Part model, mm, in its own coordinate system. A direction names the side the tool comes from. Round coordinates to 2 decimals unless told otherwise and drop trailing zeros. Order: outer loops, then holes, each group sorted by start corner. A loop starts at its lowest first (then second) coordinate and runs counter-clockwise, first axis right, second up. Notation, with made-up numbers: M 44.25,-14.75 L 66.25,-14.75 A26 cw 66.25,14.25 Z; hole C -36,-33 d4. An arc over 180 degrees is marked long. Write each question's results on one line, items separated by ' | '. Start each with the question number.
1. Band-saw the part on A-A, the plane x = 0. List the corners of the cut face in (y, z).
2. Drop flat-ended pins along their axis: pin 1 Ø3.5 at (y, z) = (-9.5, -1) entering from +X; pin 2 Ø2.5 at (x, y) = (34.43, -5) entering from +Z; pin 3 Ø0.9 at (y, z) = (-6.5, -1.5) entering from -X; pin 4 Ø8 at (x, y) = (41, 4) entering from -Z. Give the stop position or say it passes through.
3. Band-saw the part on C-C, the plane y = 16. List the corners of the cut face in (x, z).
4. Which spindle directions (+Z, -Z, +X, -X, +Y, -Y) get a long thin tool onto all of the face, cutting with end or side? Do faces 5 (the face through (44.5, 16.07, 3.54)), 6 (the face through (4.52, -13.28, -1.52)). Say none if no direction does.
5. Probe L1, parallel to Y at x = 34.43, z = 2.75; L2, parallel to Y at x = 6, z = 3.2; L3, parallel to X at y = -6, z = 5. List the from-to ranges inside material, lowest first. Write a range as [from, to].
6. Band-saw the part on B-B, the plane z = 3. Give the number of separate pieces and of enclosed holes in the cut face, then the cut area to 3 significant figures.
7. Two-plate mould, pull along X, no slides. Class faces 1 (the face through (-48, 19, 4)), 2 (the face through (50, -4, 3)), 3 (the face through (37, -4, 1)), 4 (the face through (-7, -7, 4)): +X half, -X half, draft (parallel to the pull), parting line (faces both ways), or undercut.
```python
from build123d import *

# Parameters (mm, degrees)
SKETCH_1_W                = 100
SKETCH_1_H                = 40
EXTRUDE_1_DEPTH           = 6
SKETCH_2_W                = 100
SKETCH_2_H                = 40
EXTRUDE_2_DEPTH           = 3
SKETCH_4_R                = 9.5
CUT_EXTRUDE_1_DEPTH       = 7
SKETCH_5_R                = 10.3
CUT_EXTRUDE_2_DEPTH       = 1.1
CUT_EXTRUDE_START         = -5
SKETCH_6_R                = 9.5
CUT_EXTRUDE_3_DEPTH       = 5
SKETCH_7_R                = 1.5
CUT_EXTRUDE_4_DEPTH       = 12
SKETCH_8_W                = 100
SKETCH_8_H                = 9
EXTRUDE_3_DEPTH           = 8
SKETCH_9_R                = 1.5
CUT_EXTRUDE_5_DEPTH       = 10
SKETCH_13_R               = 1.5
CUT_EXTRUDE_6_DEPTH       = 10
HOLE_WIZARD_1_D           = 3
HOLE_WIZARD_1_CBORE_D     = 5.5
HOLE_WIZARD_1_CBORE_DEPTH = 3
SKETCH_15_W               = 28
SKETCH_15_H               = 56.444719302
SKETCH_15_H_2             = 58.874458875
CUT_EXTRUDE_7_DEPTH       = 4
FILLET_3_R                = 1
FILLET_4_R                = 5
SKETCH_16_R               = 9.5
SKETCH_16_R_2             = 8.5
EXTRUDE_4_DEPTH           = 2


with BuildPart() as part:
    # 草图1 → 凸台-拉伸1 (new body)
    with BuildSketch(Plane.XY):
        Rectangle(SKETCH_1_W, SKETCH_1_H)
    extrude(amount=EXTRUDE_1_DEPTH)

    # 草图2 → 凸台-拉伸2 (add)
    with BuildSketch(Plane(origin=(0, 0, 0), x_dir=(-1, 0, 0), z_dir=(0, 0, -1))):
        Rectangle(SKETCH_2_W, SKETCH_2_H)
    extrude(amount=EXTRUDE_2_DEPTH)

    # 草图4 → 切除-拉伸1 (cut)
    with BuildSketch(Plane(origin=(0, 0, -3), x_dir=(-1, 0, 0), z_dir=(0, 0, -1))):
        Circle(SKETCH_4_R)
    extrude(amount=-CUT_EXTRUDE_1_DEPTH, mode=Mode.SUBTRACT)

    # 草图5 → 切除-拉伸2 (cut)
    with BuildSketch(Plane(origin=(0, 0, 4), x_dir=(-1, 0, 0), z_dir=(0, 0, -1))):
        Circle(SKETCH_5_R)
    extrude(amount=-CUT_EXTRUDE_2_DEPTH, mode=Mode.SUBTRACT)

    # 草图6 → 切除-拉伸3 (cut)
    with BuildSketch(Plane.XY.offset(6).offset(CUT_EXTRUDE_START)):
        with Locations(Location((0, 0, 0), (0, 0, 180))):
            Circle(SKETCH_6_R)
    extrude(amount=CUT_EXTRUDE_3_DEPTH, mode=Mode.SUBTRACT)

    # 草图7 → 切除-拉伸4 (cut)
    with BuildSketch(Plane.XY.offset(6)):
        with Locations((-15.07, 5)):
            Circle(SKETCH_7_R)
        with Locations((34.43, 5)):
            Circle(SKETCH_7_R)
        with Locations((-15.07, -5)):
            Circle(SKETCH_7_R)
        with Locations((34.43, -5)):
            Circle(SKETCH_7_R)
    extrude(amount=-CUT_EXTRUDE_4_DEPTH, mode=Mode.SUBTRACT)

    # 草图8 → 凸台-拉伸3 (add)
    with BuildSketch(Plane.XZ.offset(20)):
        with Locations((0, 1.5)):
            Rectangle(SKETCH_8_W, SKETCH_8_H)
    extrude(amount=EXTRUDE_3_DEPTH)

    # 草图9 → 切除-拉伸5 (cut)
    with BuildSketch(Plane(origin=(0, 0, -3), x_dir=(-1, 0, 0), z_dir=(0, 0, -1))):
        with Locations((-6, -15.6)):
            Circle(SKETCH_9_R)
        with Locations((6, -15.6)):
            Circle(SKETCH_9_R)
        with Locations((-16, -15.6)):
            Circle(SKETCH_9_R)
        with Locations((16, -15.6)):
            Circle(SKETCH_9_R)
    extrude(amount=-CUT_EXTRUDE_5_DEPTH, mode=Mode.SUBTRACT)

    # 草图13 → 切除-拉伸6 (cut)
    with BuildSketch(Plane.XY.offset(6)):
        with Locations((-46, 16)):
            Circle(SKETCH_13_R)
        with Locations((46, 16)):
            Circle(SKETCH_13_R)
        with Locations((-46, -24)):
            Circle(SKETCH_13_R)
        with Locations((46, -24)):
            Circle(SKETCH_13_R)
    extrude(amount=-CUT_EXTRUDE_6_DEPTH, mode=Mode.SUBTRACT)

    # 孔1 (through all)
    with Locations(Plane(origin=(-16, -15.6, -3), x_dir=(-1, 0, 0), z_dir=(0, 0, -1))):
        with Locations((0, 0), (-10, 0), (-22, 0), (-32, 0)):
            CounterBoreHole(HOLE_WIZARD_1_D / 2, HOLE_WIZARD_1_CBORE_D / 2, HOLE_WIZARD_1_CBORE_DEPTH)

    # 草图15 → 切除-拉伸7 (cut)
    with BuildSketch(Plane(origin=(0, 0, -3), x_dir=(-1, 0, 0), z_dir=(0, 0, -1))):
        with Locations((-36, -3.626193912)):
            Rectangle(SKETCH_15_W, SKETCH_15_H)
        with Locations((36, -5.588675874)):
            Rectangle(SKETCH_15_W, SKETCH_15_H_2)
    extrude(amount=-CUT_EXTRUDE_7_DEPTH, mode=Mode.SUBTRACT)

    # 圆角3
    fillet_3_edges = [part.edges().sort_by_distance(p)[0] for p in [
        (22, -4, 1),
        (-22, -4, 1),
    ]]
    fillet(fillet_3_edges, radius=FILLET_3_R)

    # 圆角4
    fillet_4_edges = [part.edges().sort_by_distance(p)[0] for p in [
        (50, -28, 3.5),
        (-50, -28, 3.5),
        (-50, 20, 3.5),
        (50, 20, 3.5),
    ]]
    fillet(fillet_4_edges, radius=FILLET_4_R)

    # 草图16 → 凸台-拉伸4 (add)
    with BuildSketch(Plane(origin=(0, 0, -3), x_dir=(-1, 0, 0), z_dir=(0, 0, -1))):
        Circle(SKETCH_16_R)
        Circle(SKETCH_16_R_2, mode=Mode.SUBTRACT)
    extrude(amount=-EXTRUDE_4_DEPTH)


solid = part.part
```
Solution:
1) outline: M -28,-3 L -8.5,-3 L -8.5,-1 L -9.5,-1 L -9.5,4 L -10.3,4 L -10.3,5.1 L -9.5,5.1 L -9.5,6 L -28,6 Z; M 8.5,-3 L 20,-3 L 20,6 L 9.5,6 L 9.5,5.1 L 10.3,5.1 L 10.3,4 L 9.5,4 L 9.5,-1 L 8.5,-1 Z
2) pin 1: x = 22.34 | pin 2: through | pin 3: x = -22 | pin 4: z = 1
3) outline: M -49.9,1 L -47.5,1 L -47.5,6 L -49.9,6 Z; M -44.5,1 L -23,1 A1 cw -22,0 L -22,-3 L 22,-3 L 22,0 A1 cw 23,1 L 44.5,1 L 44.5,6 L -44.5,6 Z; M 47.5,1 L 49.9,1 L 49.9,6 L 47.5,6 Z
4) face 5: +Z, -Z | face 6: -Z
5) L1: [-28, -6.5], [-3.5, 3.5], [6.5, 20] | L2: [-28, -17.1], [-14.1, -7.37], [7.37, 20] | L3: [-50, -16.19], [-13.95, -8.37], [8.37, 33.31], [35.55, 50]
6) separate pieces: 1 | enclosed holes: 13 | area: 4,410 mm^2
7) face 1: -X half | face 2: +X half | face 3: draft | face 4: undercut
